Part model, mm, in its own coordinate system. A direction names the side the tool comes from. Give positions to 0.01 mm unless a question says otherwise; leave off trailing zeros. Answer as a JSON object with one key per item and string values.
from build123d import *

# Parameters (mm, degrees)
SKETCH3_R          = 5.05
CUT_EXTRUDE1_DEPTH = 13
SKETCH6_R          = 6.95
CUT_EXTRUDE2_DEPTH = 8
SKETCH7_R          = 9.55
CUT_EXTRUDE3_DEPTH = 13


with BuildPart() as part:
    # Sketch1 → Revolve1 (revolve)
    with BuildSketch(Plane(origin=(0, 0, 0), x_dir=(-1, 0, 0), z_dir=(0, 0, -1))):
        with BuildLine():
            Line((-31.1, 0), (0, 0))
            Line((0, 0), (0, 12))
            Line((0, 12), (-39.6, 12))
            Line((-39.6, 12), (-40, 11.6))
            Line((-40, 11.6), (-40, 10))
            Line((-40, 10), (-45, 10))
            Line((-45, 10), (-45, 11.6))
            Line((-45, 11.6), (-45.4, 12))
            Line((-45.4, 12), (-47.1, 12))
            Line((-47.1, 12), (-47.5, 11.6))
            Line((-47.5, 11.6), (-47.5, 6.5))
            ThreePointArc((-47.5, 6.5), (-46, 5), (-47.5, 3.5))
            Line((-47.5, 3.5), (-47.5, 0.4))
            Line((-47.5, 0.4), (-47.1, 0))
            Line((-47.1, 0), (-35.4, 0))
            Line((-35.4, 0), (-35, 0.4))
            Line((-35, 0.4), (-35, 4.5))
            Line((-35, 4.5), (-31.5, 4.5))
            Line((-31.5, 4.5), (-31.5, 0.4))
            Line((-31.5, 0.4), (-31.1, 0))
        make_face()
    revolve(axis=Axis((0, 0, 0), (0, 1, 0)))

    # Sketch3 → Cut-Extrude1 (cut, through all)
    with BuildSketch(Plane(origin=(0, 12, 0), x_dir=(1, 0, 0), z_dir=(0, 1, 0))):
        with Locations((25.45, 0)):
            Circle(SKETCH3_R)
        with BuildLine():
            Line((-10.993169052, 22.409315756), (-15.964923457, 22.409315756))
            ThreePointArc((-15.964923457, 22.409315756), (-13.479046254, 15.230073041), (-10.993169052, 22.409315756))
        make_face()
        with BuildLine():
            Line((9.4402721, 24.698003254), (15.275509884, 24.698003254))
            ThreePointArc((15.275509884, 24.698003254), (18.407890992, 19.398003254), (15.275509884, 14.098003254))
            Line((15.275509884, 14.098003254), (9.4402721, 14.098003254))
            ThreePointArc((9.4402721, 14.098003254), (6.307890992, 19.398003254), (9.4402721, 24.698003254))
        make_face()
        with BuildLine():
            Line((-10.993169052, -22.409315756), (-15.964923457, -22.409315756))
            ThreePointArc((-15.964923457, -22.409315756), (-13.479046254, -15.230073041), (-10.993169052, -22.409315756))
        make_face()
        with BuildLine():
            Line((9.4402721, -14.098003254), (15.275509884, -14.098003254))
            ThreePointArc((15.275509884, -14.098003254), (18.407890992, -19.398003254), (15.275509884, -24.698003254))
            Line((15.275509884, -24.698003254), (9.4402721, -24.698003254))
            ThreePointArc((9.4402721, -24.698003254), (6.307890992, -19.398003254), (9.4402721, -14.098003254))
        make_face()
    extrude(amount=-CUT_EXTRUDE1_DEPTH, mode=Mode.SUBTRACT)

    # Sketch6 → Cut-Extrude2 (cut)
    with BuildSketch(Plane(origin=(0, 0, 0), x_dir=(-1, 0, 0), z_dir=(0, -1, 0))):
        with Locations((13.479046254, 19.250073041)):
            Circle(SKETCH6_R)
        with Locations((13.479046254, -19.250073041)):
            Circle(SKETCH6_R)
    extrude(amount=-CUT_EXTRUDE2_DEPTH, mode=Mode.SUBTRACT)

    # Sketch7 → Cut-Extrude3 (cut, through all)
    with BuildSketch(Plane(origin=(0, 12, 0), x_dir=(1, 0, 0), z_dir=(0, 1, 0))):
        Circle(SKETCH7_R)
    extrude(amount=-CUT_EXTRUDE3_DEPTH, mode=Mode.SUBTRACT)


solid = part.part
1. Cut at A-A on y = 2. State how many separate pieces and enclosed holes the cut face has, plus the area to 3 significant figures.
Worked answers:
{"separate pieces": "2", "enclosed holes": "7", "area": "5,470 mm^2"}
2. Which spindle directions (+Z, -Z, +X, -X, +Y, -Y) get a long thin tool onto all of the face, cutting with end or side? Do faces 1 (the cylindrical face through (20.765, 10.811, 39.923)), 2 (the cylindrical face through (-4.101, 2.421, -31.232)), 3 (the flat face through (-13, 10, -22.409)). Say none if no direction does.
Worked answers:
{"face 1": "+Y", "face 2": "-Y", "face 3": "+Y, -Y"}
3. Probe line 1 along X through (y, z) = (9.5, 0); line 2 along X through (y, z) = (1.75, -23); line 3 along Z through (x, y) = (0, 10.55). List the from-to ranges inside material, lowest first.
Worked answers:
{"line 1": "x = -47.5 to -9.55, 9.55 to 20.4, 30.5 to 47.5", "line 2": "x = -41.56 to -26.38, -21.52 to -19.33, -7.63 to 7.5, 17.22 to 21.52, 26.38 to 41.56", "line 3": "z = -47.5 to -45, -40 to -9.55, 9.55 to 40, 45 to 47.5"}
4. Pin check, flat tips, straight feed: P1, Ø1.5, axis at y = 3, z = 27.5, coming from the -X side; P2, Ø13, axis at x = -13.48, z = -19.25, coming from the -Y side; P3, Ø6.5, axis at x = 12.5, y = 5.5, coming from the -Z side. Stop position of each tip, or through.
Worked answers:
{"P1": "stops at x = -39.25", "P2": "stops at y = 8", "P3": "stops at z = -46.56"}
5. Two-plate mould, pull along X, no slides. Class faces 4 (the cylindrical face through (-10.3, 9.01, 46.37)), 5 (the flat face through (25, 12, -39)), 6 (the cylindrical face through (-13.618, 10.028, 15.232)): +X half, -X half, draft (parallel to the pull), parting line (faces both ways), or undercut.
Worked answers:
{"face 4": "parting line", "face 5": "draft", "face 6": "undercut"}
